Part model, mm, in its own coordinate system. A direction names the side the tool comes from. Give positions to 0.01 mm unless a question says otherwise; leave off trailing zeros. Order: outer loops, then holes, each group sorted by start corner. A loop starts at its lowest first (then second) coordinate and runs counter-clockwise, first axis right, second up. Notation, with made-up numbers: (14, -15.5) - (34, -15.5) arc R15 cw to (34, 2.5) - close; hole circle Ø1 at (14.25, 46.25). An arc over 180 degrees is marked (long way). Use a Markdown table: item, result. Add a question column.
from build123d import *

# Parameters (mm, degrees)
BOSS_EXTRU_1_DEPTH      = 25.52
ESQUISSE2_R             = 6.325
ENL_V_MAT_EXTRU_1_DEPTH = 1.75
ESQUISSE3_R             = 1.5
ENL_V_MAT_EXTRU_2_DEPTH = 25.52
ESQUISSE6_W             = 3
ESQUISSE6_H             = 51
BOSS_EXTRU_2_DEPTH      = 17
CONG_1_R                = 2
CONG_2_R                = 1
ESQUISSE7_R             = 1.5
ENL_V_MAT_EXTRU_3_DEPTH = 29.52
CONG_3_R                = 5
ESQUISSE8_R             = 1.5
ENL_V_MAT_EXTRU_4_DEPTH = 18


with BuildPart() as part:
    # Esquisse1 → Boss.-Extru.1 (new body)
    with BuildSketch(Plane(origin=(0, 0, 0), x_dir=(0, 0, -1), z_dir=(1, 0, 0))):
        with BuildLine():
            Line((0, 27), (0, 5))
            ThreePointArc((0, 5), (1.464466094, 1.464466094), (5, 0))
            Line((5, 0), (80.5, 0))
            ThreePointArc((80.5, 0), (84.035533906, 1.464466094), (85.5, 5))
            Line((85.5, 5), (85.5, 27))
            Line((85.5, 27), (83.75, 27))
            Line((83.75, 27), (83.75, 5))
            ThreePointArc((83.75, 5), (82.798097039, 2.701902961), (80.5, 1.75))
            Line((80.5, 1.75), (5, 1.75))
            ThreePointArc((5, 1.75), (2.701902961, 2.701902961), (1.75, 5))
            Line((1.75, 5), (1.75, 27))
            Line((1.75, 27), (0, 27))
        make_face()
    extrude(amount=BOSS_EXTRU_1_DEPTH)

    # Esquisse2 → Enlèv. mat.-Extru.1 (cut)
    with BuildSketch(Plane.XY):
        with Locations((12.76, 17.25)):
            Circle(ESQUISSE2_R)
    extrude(amount=-ENL_V_MAT_EXTRU_1_DEPTH, mode=Mode.SUBTRACT)

    # Esquisse3 → Enlèv. mat.-Extru.2 (cut)
    with BuildSketch(Plane(origin=(0, 0, -85.5), x_dir=(-1, 0, 0), z_dir=(0, 0, -1))):
        with Locations((-12.76, 17.25)):
            Circle(ESQUISSE3_R)
    extrude(amount=-ENL_V_MAT_EXTRU_2_DEPTH, mode=Mode.SUBTRACT)

    # Esquisse6 → Boss.-Extru.2 (add)
    with BuildSketch(Plane(origin=(0, 1.75, 0), x_dir=(1, 0, 0), z_dir=(0, 1, 0))):
        with Locations((27.02, 42.75)):
            Rectangle(ESQUISSE6_W, ESQUISSE6_H)
    extrude(amount=-BOSS_EXTRU_2_DEPTH)

    # Congé1
    cong_1_edges = [part.edges().sort_by_distance(p)[0] for p in [
        (28.52, 1.75, -42.75),
    ]]
    fillet(cong_1_edges, radius=CONG_1_R)

    # Congé2
    cong_2_edges = [part.edges().sort_by_distance(p)[0] for p in [
        (25.52, 0, -42.75),
    ]]
    fillet(cong_2_edges, radius=CONG_2_R)

    # Esquisse7 → Enlèv. mat.-Extru.3 (cut, through all)
    with BuildSketch(Plane(origin=(28.52, 0, 0), x_dir=(0, 0, -1), z_dir=(1, 0, 0))):
        with Locations((23.25, -7.75)):
            Circle(ESQUISSE7_R)
        with Locations((62.25, -7.75)):
            Circle(ESQUISSE7_R)
    extrude(amount=-ENL_V_MAT_EXTRU_3_DEPTH, mode=Mode.SUBTRACT)

    # Congé3
    cong_3_edges = [part.edges().sort_by_distance(p)[0] for p in [
        (27.02, -15.25, -68.25),
        (27.02, -15.25, -17.25),
    ]]
    fillet(cong_3_edges, radius=CONG_3_R)

    # Esquisse8 → Enlèv. mat.-Extru.4 (cut, through all)
    with BuildSketch(Plane(origin=(0, 1.75, 0), x_dir=(1, 0, 0), z_dir=(0, 1, 0))):
        with Locations((20.01, 49.45)):
            Circle(ESQUISSE8_R)
        with Locations((5.51, 49.45)):
            Circle(ESQUISSE8_R)
    extrude(amount=-ENL_V_MAT_EXTRU_4_DEPTH, mode=Mode.SUBTRACT)


solid = part.part
1. Cut at B-B (x = 12.76). Write the cut outline in (y, z) (3 decimals), plus the area to 3 significant figures.
2. Tool access for faces 1 (the face through (12.581, 2.677, -2.727)), 2 (the face through (15, 11, 0)): list every direction of +Z, -Z, +X, -X, +Y, -Y with a clear straight run to the whole face (end or side of a thin tool).
3. Mould opens along X. For faces 3 (the face through (27.041, -8.325, -63.636)), 4 (the face through (11.954, 18.515, -84.637)), 5 (the face through (27.95, 1.15, -43.11)) say: released by +X, released by -X, zero draft, split by the parting line, or undercut.
4. Pin check, flat tips, straight feed: P1, Ø2.5, axis at y = -7.75, z = -23.25, coming from the +X side; P2, Ø4, axis at y = -7.75, z = -62.25, coming from the -X side; P3, Ø1, axis at x = 12.5, y = 21.5, coming from the +Z side; P4, Ø2, axis at x = 27, y = -2.5, coming from the +Z side. Stop position of each tip, or through.
5. Cut at D-D (z = -23.25). Write the cut outline in (x, y), plus the area to 3 significant figures.
6. Cut at A-A (z = -49.45). Write the cut outline in (x, y).
7. Cut at C-C (x = 20.01). Write the cut outline in (y, z).
8. Drill centre lines: probe 1 along X at (y, z) = (0.8, -49.45); probe 2 along X at (y, z) = (0.6, -49.45); probe 3 along Y at (x, z) = (26.4, -62.25). Where is each one in solid material? Low to high. Write a range as [from, to].
Responses:
| question | item | result |
|---|---|---|
| 1 | outline | (0, -80.5) arc R5 ccw to (5, -85.5) - (15.75, -85.5) - (15.75, -83.75) - (5, -83.75) arc R3.25 cw to (1.75, -80.5) - (1.75, -5) arc R3.25 cw to (5, -1.75) - (10.925, -1.75) - (10.925, 0) - (5, 0) arc R5 ccw to (0, -5) - close; (18.75, -85.5) - (27, -85.5) - (27, -83.75) - (18.75, -83.75) - close; (23.575, -1.75) - (27, -1.75) - (27, 0) - (23.575, 0) - close |
| 1 | area | 204 mm² |
| 2 | face 1 | +X, -X, +Y |
| 2 | face 2 | +Z, +X, -X, +Y, -Y |
| 3 | face 3 | zero draft |
| 3 | face 4 | undercut |
| 3 | face 5 | released by +X |
| 4 | P1 | passes through |
| 4 | P2 | stops at x = 25.52 |
| 4 | P3 | stops at z = -83.75 |
| 4 | P4 | stops at z = -17.25 |
| 5 | outline | (0, 0) - (24.52, 0) arc R1 cw to (25.52, -1) - (25.52, -6.25) - (28.52, -6.25) - (28.52, -0.25) arc R2 ccw to (26.52, 1.75) - (0, 1.75) - close; (25.52, -15.25) - (28.52, -15.25) - (28.52, -9.25) - (25.52, -9.25) - close |
| 5 | area | 86.0 mm² |
| 6 | outline | (0, 0) - (4.01, 0) - (4.01, 1.75) - (0, 1.75) - close; (7.01, 0) - (18.51, 0) - (18.51, 1.75) - (7.01, 1.75) - close; (21.51, 0) - (24.52, 0) arc R1 cw to (25.52, -1) - (25.52, -15.25) - (28.52, -15.25) - (28.52, -0.25) arc R2 ccw to (26.52, 1.75) - (21.51, 1.75) - close |
| 7 | outline | (0, -80.5) arc R5 ccw to (5, -85.5) - (27, -85.5) - (27, -83.75) - (5, -83.75) arc R3.25 cw to (1.75, -80.5) - (1.75, -50.95) - (0, -50.95) - close; (0, -47.95) - (1.75, -47.95) - (1.75, -5) arc R3.25 cw to (5, -1.75) - (27, -1.75) - (27, 0) - (5, 0) arc R5 ccw to (0, -5) - close |
| 8 | probe 1 | x = [0, 4.01], [7.01, 18.51], [21.51, 28.22] |
| 8 | probe 2 | x = [0, 4.01], [7.01, 18.51], [21.51, 28.33] |
| 8 | probe 3 | y = [-15.25, -9.25], [-6.25, 1.75] |
